Job drawing, mm, ordinate dimensions from the low corner. One solid piece. Give positions to 0.01 mm unless a question says otherwise; leave off trailing zeros. Write each loop counter-clockwise with the first axis right and the second up, starting at its lowest first coordinate (ties: lowest second). Pieces come first, ordered by that corner, then holes. Notation, with made-up numbers: M 63.5,8 L 91.5,8 A27 cw 91.5,47 Z; hole C 22.5,-2 d8. An arc over 180 degrees is marked long. Use CSV: the item, a comma, the result in double quotes. Start each with the question number.
Item 1: Drill centre lines: line 1 (Y direction, x = 70, z = 4.05); line 2 (Y direction, x = 50, z = 4.5); line 3 (X direction, y = 105, z = 4.5). Where is each one in solid material? Low to high. Write a range as [from, to].
Item 2: Cut at D-D (y = 62.5). List the corners of the cut face in (x, z), then the cut area to 3 significant figures.
Item 3: Cut at B-B (x = 110). List the corners of the cut face in (y, z), then the cut area to 3 significant figures.
Item 4: Cut at A-A (x = 50). List the corners of the cut face in (y, z), then the cut area to 3 significant figures.
Item 5: Cut at C-C (z = 3.25). List the corners of the cut face in (x, y), then the cut area to 3 significant figures.
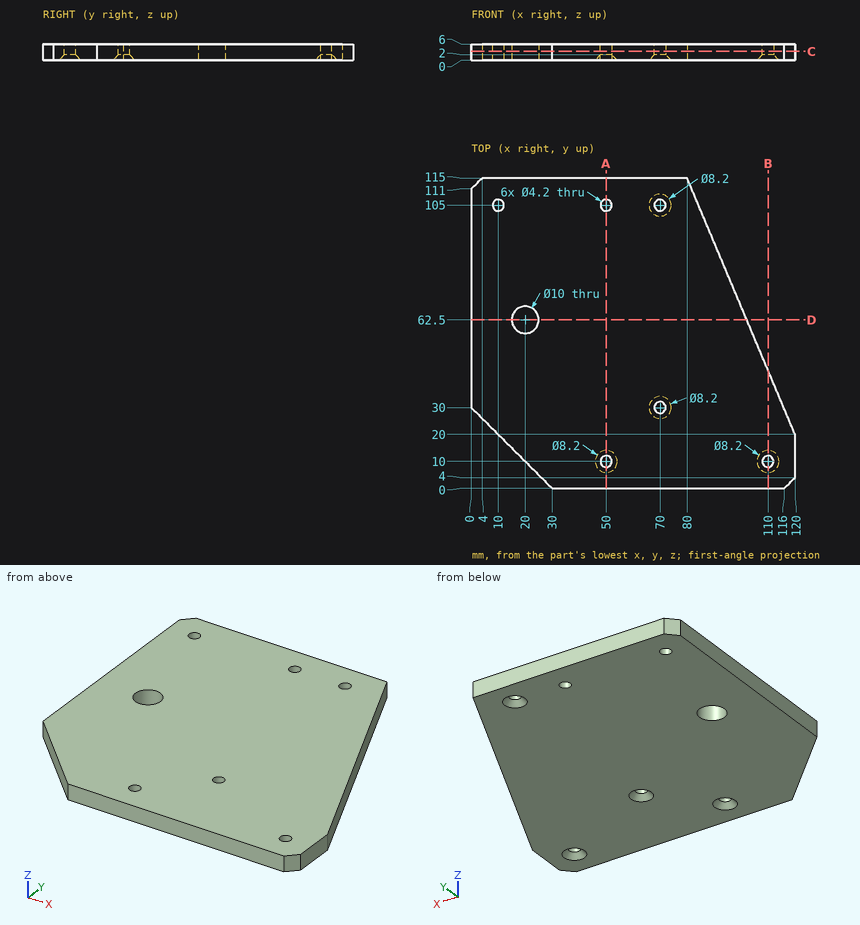
Worked answers:
1,line 1,"y = [0, 27.9], [32.1, 102.9], [107.1, 115]"
1,line 2,"y = [0, 7.9], [12.1, 102.9], [107.1, 115]"
1,line 3,"x = [0, 7.9], [12.1, 47.9], [52.1, 67.9], [72.1, 84.21]"
2,outline,"M 0,0 L 15,0 L 15,6 L 0,6 Z; M 25,0 L 102.11,0 L 102.11,6 L 25,6 Z"
2,area,"553 mm^2"
3,outline,"M 0,0 L 5.9,0 L 7.9,2 L 7.9,6 L 0,6 Z; M 12.1,2 L 14.1,0 L 43.75,0 L 43.75,6 L 12.1,6 Z"
3,area,"233 mm^2"
4,outline,"M 0,0 L 5.9,0 L 7.9,2 L 7.9,6 L 0,6 Z; M 12.1,2 L 14.1,0 L 102.9,0 L 102.9,6 L 12.1,6 Z; M 107.1,0 L 115,0 L 115,6 L 107.1,6 Z"
4,area,"636 mm^2"
5,outline,"M 0,30 L 30,0 L 116,0 L 120,4 L 120,20 L 80,115 L 4,115 L 0,111 Z; hole C 10,105 d4.2; hole C 20,62.5 d10; hole C 50,10 d4.2; hole C 50,105 d4.2; hole C 70,30 d4.2; hole C 70,105 d4.2; hole C 110,10 d4.2"
5,area,"11,300 mm^2"
